Here's the drawing with two shaded views (mm, measured from the low corner). I have some questions. Coordinates: 2 decimals unless noted, no trailing zeros. Loops run counter-clockwise (first coordinate to the right, second up) from the corner with the lowest first, then second, coordinate; pieces in that order, holes last. Notation, with made-up numbers: (20, 46.5) - (72, 46.5) arc R28 cw to (72, 81.5) - close; hole circle Ø7 at (-10, 23). An arc over 180 degrees is marked (long way). Use a Markdown table: item, result.
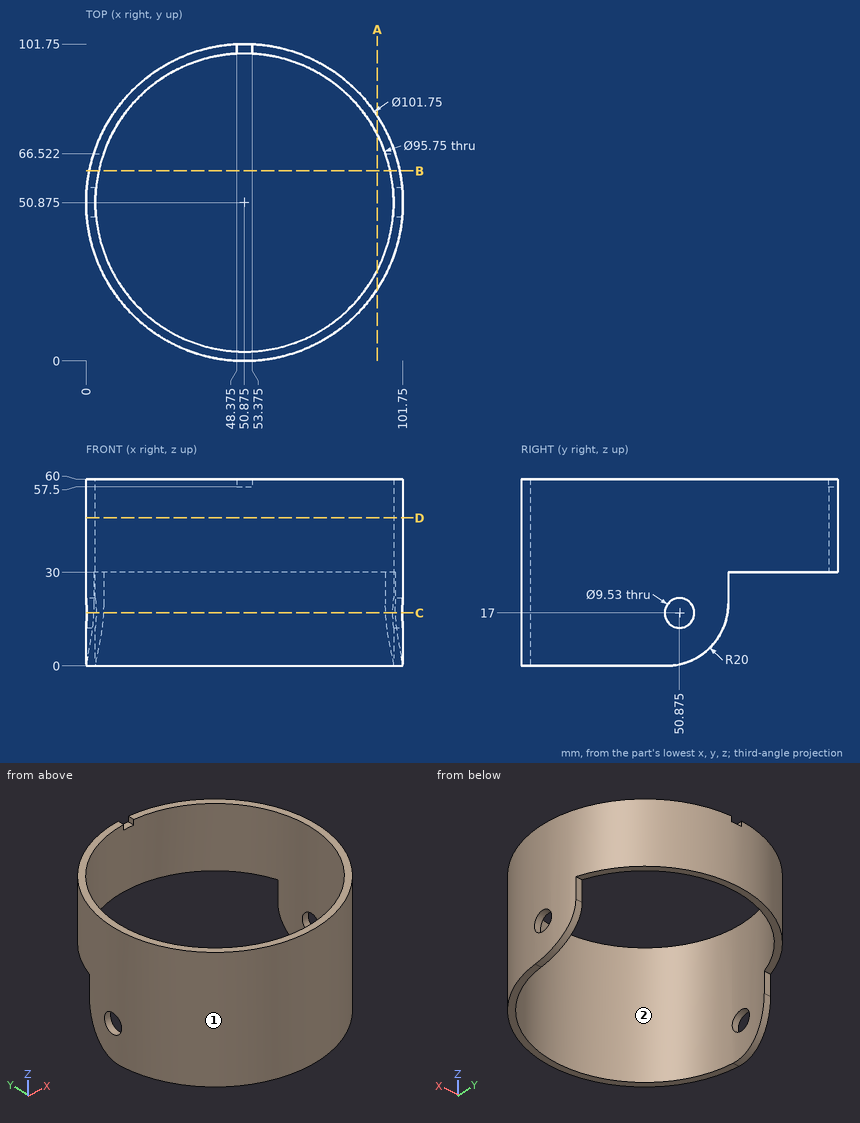
Q1. I want a section at C-C, the plane z = 17. Give the number of separate pieces and of enclosed holes in the cut face, then the cut area to 3 significant figures.
Check values:
| item | result |
|---|---|
| separate pieces | 3 |
| enclosed holes | 0 |
| area | 502 mm^2 |
Q2. I want a section at B-B, the plane y = 61. Write out the boundary of the cut face in (x, z), then the cut area to 3 significant figures.
Check values:
| item | result |
|---|---|
| outline | (1.02, 6.2) - (4.08, 6.2) - (4.08, 60) - (1.02, 60) - close; (97.67, 6.2) - (100.73, 6.2) - (100.73, 60) - (97.67, 60) - close |
| area | 330 mm^2 |
Q3. I want a section at D-D, the plane z = 47.5. Write out the boundary of the cut face in (x, y) (3 decimals), then the cut area to 3 significant figures.
Check values:
| item | result |
|---|---|
| outline | circle Ø101.75 at (50.875, 50.875); hole circle Ø95.75 at (50.875, 50.875) |
| area | 931 mm^2 |
Q4. I want a section at A-A, the plane x = 93.5. Write out the boundary of the cut face in (y, z).
Check values:
| item | result |
|---|---|
| outline | (23.1, 0) - (29.08, 0) - (29.08, 60) - (23.1, 60) - close; (72.67, 30) - (78.65, 30) - (78.65, 60) - (72.67, 60) - close |
Q5. Will these pins go through, and if not, where does the flat tip stop? P1, Ø10, axis at x = 27.5, z = 31.5, coming from the -Y side; P2, Ø1.5, axis at x = 14.5, z = 47, coming from the +Y side (1 decimal); P3, Ø1.5, axis at x = 50, y = 100.5, coming from the +Z side; P4, Ø5.5, axis at y = 50.875, z = 17, coming from the +X side.
Check values:
| item | result |
|---|---|
| P1 | y = 3.43 |
| P2 | y = 87.2 |
| P3 | z = 57.5 |
| P4 | through |
Q6. Please list where these lines run through material, in increasing order: L1, parallel to X at y = 50, z = 44; L2, parallel to X at y = 8.5, z = 7 (1 decimal); L3, parallel to Y at x = 80, z = 49.5. Write a range as from..to.
Check values:
| item | result |
|---|---|
| L1 | 0.01..3.01, 98.74..101.74 |
| L2 | 22.7..28.6, 73.2..79 |
| L3 | 9.16..12.88, 88.87..92.59 |
Q7. If we mould it in two halves opening along Y, with no side actions, what happens to the marked faces 1 and 2? For each: pulls with the +Y half, pulls with the -Y half, needs draft (parallel to the pull), parting line crosses it, or undercut.
Check values:
| item | result |
|---|---|
| face 1 | parting line crosses it |
| face 2 | undercut |
